```python
from build123d import *

# Parameters (mm, degrees)
SKIZZE1_W   = 160
SKIZZE1_H   = 5
SKIZZE1_W_2 = 100


with BuildPart() as part:
    # Skizze1 → Rotation1 (revolve)
    with BuildSketch(Plane.XY, mode=Mode.PRIVATE) as rotation1_sk:
        with Locations((80, 77.5)):
            Rectangle(SKIZZE1_W, SKIZZE1_H)
        with Locations((160, 72.5)):
            Rectangle(SKIZZE1_W_2, SKIZZE1_H)
    revolve(rotation1_sk.sketch.rotate(Axis((0, 0, 0), (1, 0, 0)), 90), axis=Axis((0, 0, 0), (1, 0, 0)))


solid = part.part
```
Design review of the part built by this model. Coordinates are the model's own, in mm. A direction names the side the tool comes from. Coordinates: 2 decimals unless noted, no trailing zeros. Write each loop counter-clockwise with the first axis right and the second up, starting at its lowest first coordinate (ties: lowest second). Pieces come first, ordered by that corner, then holes.
1) Add section D-D (x = 71.5). Write out the cut boundary in (y, z), plus the area to 3 significant figures.
2) Machinability: for faces 4 (the cylindrical face through (185.35, 66.538, 34.608)), 5 (the flat face through (210, 50, -50)), 6 (the cylindrical face through (55.77, 66.538, 34.608)), which of the approach directions +Z, -Z, +X, -X, +Y, -Y give a long, thin tool a straight path to every point of the face, cutting with its end or side? Answer none if there is none.
3) Add section C-C (x = 187.5). Write out the cut boundary in (y, z), plus the area to 3 significant figures.
4) Add section A-A (y = 0). Write out the cut boundary in (x, z).
5) Insertion check: pin 1 (4 mm diameter, centred on x = 114, z = 52, fed in from +Y); pin 2 (10 mm diameter, centred on x = 44, y = 14, fed in from -Z); pin 3 (1 mm diameter, centred on y = -47.5, z = 57, fed in from -X). Each pin has a flat end and moves straight along its axis. Give the tip position at first contact, or say it passes through.
6) To check wall thickness, follow L1, parallel to Y at x = 70, z = 0; L2, parallel to Y at x = 189, z = 0; L3, parallel to Z at x = 64, y = -11.5. State the ranges of each line that lie inside material, in increasing order.
7) Mouldability with a two-part tool opening along Z and no side actions: class faces 1 (the flat face through (0, -71.5, -23.3)), 2 (the flat face through (110, 50, -50)), 3 (the cylindrical face through (81.12, -3.517, -79.923)) as +Z half, -Z half, draft (parallel to the pull), parting line (faces both ways), or undercut.
Check result:
1. outline: circle Ø160 at (0, 0); hole circle Ø150 at (0, 0)
1. area: 2,430 mm2
2. face 4: +X
2. face 5: +Z, -Z, +X, +Y, -Y
2. face 6: -X
3. outline: circle Ø150 at (0, 0); hole circle Ø140 at (0, 0)
3. area: 2,280 mm2
4. outline: (0, -80) - (160, -80) - (160, -75) - (210, -75) - (210, -70) - (110, -70) - (110, -75) - (0, -75) - close; (0, 75) - (110, 75) - (110, 70) - (210, 70) - (210, 75) - (160, 75) - (160, 80) - (0, 80) - close
5. pin 1: stops at y = 62.45
5. pin 2: stops at z = -79.49
5. pin 3: stops at x = 110
6. L1: y = -80 to -75, 75 to 80
6. L2: y = -75 to -70, 70 to 75
6. L3: z = -79.17 to -74.11, 74.11 to 79.17
7. face 1: draft
7. face 2: undercut
7. face 3: parting line
